Design review of the part shown in the three views and the two pictorial views. Dimensions are in mm from the part's minimum x, y and z. A direction names the side the tool comes from. Give positions to 0.01 mm unless a question says otherwise; leave off trailing zeros. Order: outer loops, then holes, each group sorted by start corner. A loop starts at its lowest first (then second) coordinate and runs counter-clockwise, first axis right, second up.
Item 1: For probe 1 along Y at (x, z) = (7, 1.85); probe 2 along Y at (x, z) = (6, 2.1); probe 3 along Y at (x, z) = (3, 2.85), list the stretches that pass through material, from the lowest coordinate up.
Item 2: Consider section C-C (z = 2.7). Give the boundary of the cut face in (x, y), plus the area to 3 significant figures.
Item 3: Consider section B-B (y = 15). Give the boundary of the cut face in (x, z), plus the area to 3 significant figures.
Item 4: The part is to be moulded in two halves that separate along Y. For the marked faces 3, 4, 5 and 6, say which applies: released by +Y, released by -Y, zero draft, split by the parting line, or undercut.
Item 5: Machinability: for the marked faces 1 and 2, which of the approach directions +Z, -Z, +X, -X, +Y, -Y give a long, thin tool a straight path to every point of the face, cutting with its end or side? Answer none if there is none.
Item 6: Consider section A-A (x = 7). Give the boundary of the cut face in (y, z).
Item 7: Consider section D-D (y = 24.25). Give the boundary of the cut face in (x, z), plus the area to 3 significant figures.
Item 8: For P1, Ø0.9, axis at x = 7.5, z = 1, coming from the -Y side, flat-tipped, find the tip position at first contact; note if it passes through.
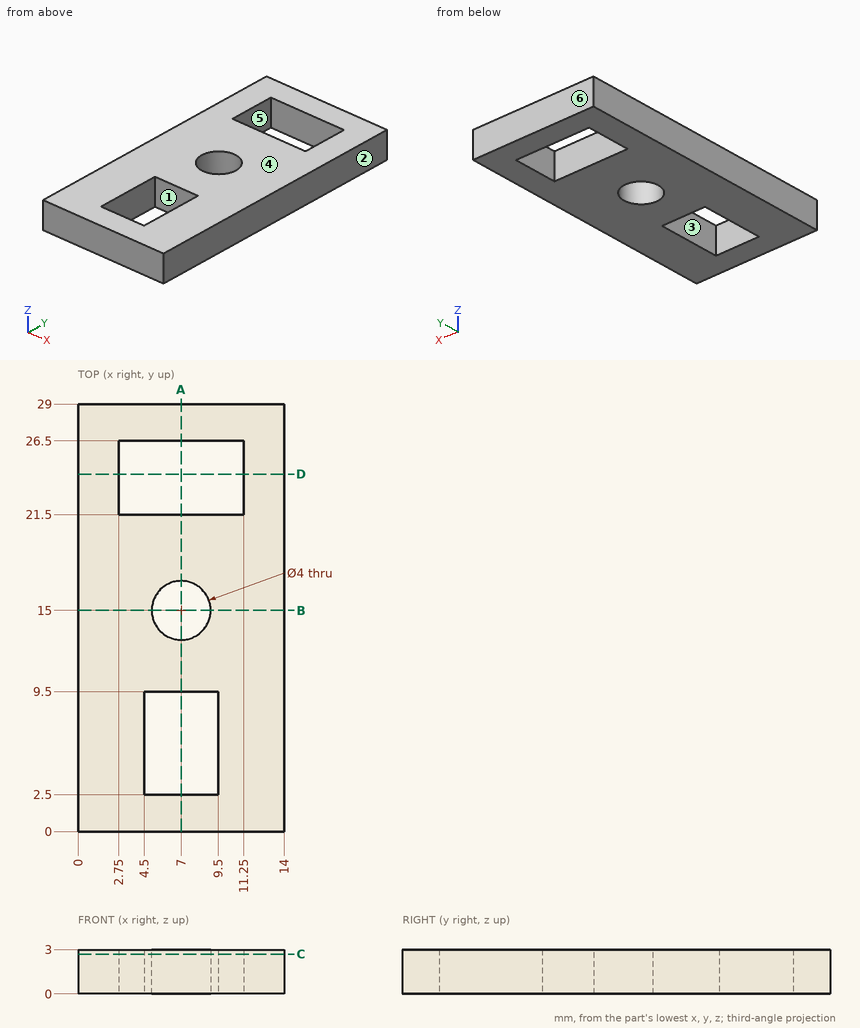
Resolved:
1. probe 1: y = 0 to 2.5, 9.5 to 13, 17 to 21.5, 26.5 to 29
1. probe 2: y = 0 to 2.5, 9.5 to 13.27, 16.73 to 21.5, 26.5 to 29
1. probe 3: y = 0 to 21.5, 26.5 to 29
2. outline: (0, 0) - (14, 0) - (14, 29) - (0, 29) - close; hole (2.75, 21.5) - (11.25, 21.5) - (11.25, 26.5) - (2.75, 26.5) - close; hole (4.5, 2.5) - (9.5, 2.5) - (9.5, 9.5) - (4.5, 9.5) - close; hole circle Ø4 at (7, 15)
2. area: 316 mm2
3. outline: (0, 0) - (5, 0) - (5, 3) - (0, 3) - close; (9, 0) - (14, 0) - (14, 3) - (9, 3) - close
3. area: 30.0 mm2
4. face 3: undercut
4. face 4: zero draft
4. face 5: undercut
4. face 6: released by +Y
5. face 1: +Z, -Z
5. face 2: +Z, -Z, +X, +Y, -Y
6. outline: (0, 0) - (2.5, 0) - (2.5, 3) - (0, 3) - close; (9.5, 0) - (13, 0) - (13, 3) - (9.5, 3) - close; (17, 0) - (21.5, 0) - (21.5, 3) - (17, 3) - close; (26.5, 0) - (29, 0) - (29, 3) - (26.5, 3) - close
7. outline: (0, 0) - (2.75, 0) - (2.75, 3) - (0, 3) - close; (11.25, 0) - (14, 0) - (14, 3) - (11.25, 3) - close
7. area: 16.5 mm2
8. P1: stops at y = 0
